Study the drawing (mm; zero at the part's minimum x, y, z) and answer. A direction names the side the tool comes from. Round coordinates to 2 decimals unless told otherwise and drop trailing zeros. Write each loop counter-clockwise with the first axis right and the second up, starting at its lowest first coordinate (ties: lowest second). Pieces come first, ordered by that corner, then holes.
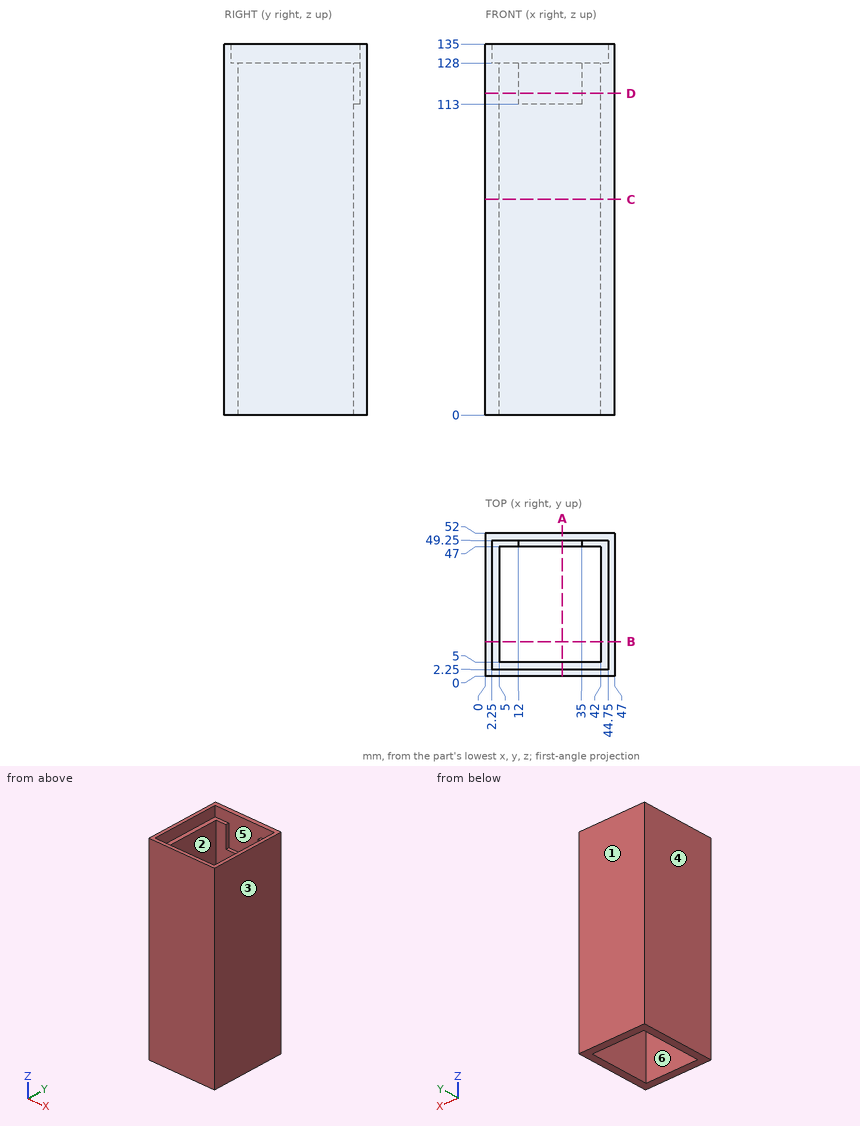
Q1. Given pin 1 (13 mm diameter, centred on x = 17.5, y = 28, fed in from +Z), flat-ended and moving along its own axis, determine where the tip first touches the part or whether it passes through.
Q2. Find section C-C (z = 78.5). Determine the outline of the cut face in (x, y).
Q3. Find section D-D (z = 117). Determine the outline of the cut face in (x, y).
Q4. Find section A-A (x = 28). Determine the outline of the cut face in (y, z).
Q5. Find the intervals of material crossed by L1, parallel to X at y = 7.5, z = 124; L2, parallel to Y at x = 30, z = 66.5; L3, parallel to Y at x = 20.5, z = 122, in increasing order.
Q6. The mould has two halves that part along X. Classify the marked faces 1, 2 and 3: +X half, -X half, draft (parallel to the pull), parting line (faces both ways), or undercut.
Q7. Find section B-B (y = 12.5). Determine the outline of the cut face in (x, z).
Q8. A tool of negligible diameter and unlimited length cuts with its end or side. For the marked faces 4, 5 and 6, from which of +Z, -Z, +X, -X, +Y, -Y can it reach the whole face along a straight path? Write none if from no direction.
Report:
1. pin 1: passes through
2. outline: (0, 0) - (47, 0) - (47, 52) - (0, 52) - close; hole (5, 5) - (42, 5) - (42, 47) - (5, 47) - close
3. outline: (0, 0) - (47, 0) - (47, 52) - (0, 52) - close; hole (5, 5) - (42, 5) - (42, 47) - (35, 47) - (35, 49.25) - (12, 49.25) - (12, 47) - (5, 47) - close
4. outline: (0, 0) - (5, 0) - (5, 128) - (2.25, 128) - (2.25, 135) - (0, 135) - close; (47, 0) - (52, 0) - (52, 135) - (49.25, 135) - (49.25, 113) - (47, 113) - close
5. L1: x = 0 to 5, 42 to 47
5. L2: y = 0 to 5, 47 to 52
5. L3: y = 0 to 5, 49.25 to 52
6. face 1: draft
6. face 2: undercut
6. face 3: +X half
7. outline: (0, 0) - (5, 0) - (5, 128) - (2.25, 128) - (2.25, 135) - (0, 135) - close; (42, 0) - (47, 0) - (47, 135) - (44.75, 135) - (44.75, 128) - (42, 128) - close
8. face 4: +Z, -Z, -X, +Y, -Y
8. face 5: +Z
8. face 6: +Z, -Z
